Design review of the part built by this model. Coordinates are the model's own, in mm. Face numbers are marked on the shaded views. Round coordinates to 2 decimals unless told otherwise and drop trailing zeros. Order: outer loops, then holes, each group sorted by start corner. A loop starts at its lowest first (then second) coordinate and runs counter-clockwise, first axis right, second up. Notation, with made-up numbers: M 35.25,50 L 92.25,50 A18 cw 92.25,54 Z; hole C -6,6.25 d4. An arc over 180 degrees is marked long. Write each question's results on one line, items separated by ' | '. Start each with the question number.
Item 1: Take a section at B-B, the plane y = 20. Write out the cut boundary in (x, z).
Item 2: Take a section at A-A, the plane x = 0. Write out the cut boundary in (y, z), plus the area to 3 significant figures.
Item 3: Clearance check with flat-ended pins moving along their axes: pin 1 (2 mm diameter, centred on y = 40.5, z = 7.5, fed in from +X); pin 2 (1.9 mm diameter, centred on x = 6.23, y = 33.21, fed in from -Z); pin 3 (3.5 mm diameter, centred on x = -4.33, y = 27.5, fed in from -Z); pin 4 (6 mm diameter, centred on y = 7.5, z = 6, fed in from +X). State where each tip first meets the part, or that it passes through.
Item 4: The part is to be moulded in two halves that separate along Z. For the marked faces 1, 2 and 3, say which applies: +Z half, -Z half, draft (parallel to the pull), parting line (faces both ways), or undercut.
Item 5: Wall thickness on line 1 (Y direction, x = -4, z = 3); line 2 (Y direction, x = 0, z = 5.05); line 3 (Z direction, x = 21.5, y = 20.5): over which ranges is each line inside the solid? List them lowest first. Write a range as [from, to].
Item 6: Take a section at C-C, the plane z = 12.25. Write out the cut boundary in (x, y), plus the area to 3 significant figures.
Item 7: Take a section at D-D, the plane y = 36. Count the separate pieces of the cut face and the enclosed holes in it, plus the area to 3 significant figures.
```python
from build123d import *

# Parameters (mm, degrees)
SKETCH_1_R               = 27.5
EXTRUDE_1_DEPTH          = 6
SKETCH_2_R               = 6
SKETCH_2_R_2             = 3.499999999999999
EXTRUDE_2_DEPTH          = 6
PATTERN_CIRCULAR_3_COUNT = 3
CUT_EXTRUDE_1_DEPTH      = 61.37176492367935
FILLET_1_R               = 10
SKETCH_6_R               = 1.6000000000000016
SKETCH_6_R_2             = 1.6
CUT_EXTRUDE_2_DEPTH      = 62.79603560803595
SKETCH_7_R               = 2.999999999999999
CUT_EXTRUDE_3_DEPTH      = 61.37176506339406
PATTERN_CIRCULAR_4_COUNT = 3
SKETCH_8_R               = 1.5000000000000009
SKETCH_8_R_2             = 1.5000000000000018
SKETCH_8_R_3             = 1.5
CUT_EXTRUDE_4_DEPTH      = 61.37176506339406
FILLET_2_R               = 1


with BuildPart() as part:
    # 草图1 → 凸台-拉伸1 (new body)
    with BuildSketch(Plane.XY):
        with Locations((0, 25)):
            Circle(SKETCH_1_R)
    extrude(amount=EXTRUDE_1_DEPTH)

    # 草图2 → 凸台-拉伸2 (add)
    with BuildSketch(Plane(origin=(0, 0, 0), x_dir=(1, 0, 0), z_dir=(0, 1, 0))):
        with Locations((0, -11.5)):
            Circle(SKETCH_2_R)
        with Locations(Location((0, -11.5, 0), (0, 0, 270))):
            Circle(SKETCH_2_R_2, mode=Mode.SUBTRACT)
    extrude_2 = extrude(amount=EXTRUDE_2_DEPTH)

    # 阵列(圆周)3: 凸台-拉伸2 ×3 about axis
    pattern_circular_3_axis = Axis((8.33e-15, 25.000000000000004, 0), (0, 0, 1))
    for i in range(1, PATTERN_CIRCULAR_3_COUNT):
        add(extrude_2.rotate(pattern_circular_3_axis, i * 360 / PATTERN_CIRCULAR_3_COUNT))

    # 草图5 → 切除-拉伸1 (cut, through all)
    with BuildSketch(Plane.XY.offset(6)):
        with BuildLine():
            Line((-20.45167721378295, 39.57665596572934), (-15.92241547591627, 47.42156741649214))
            ThreePointArc((-15.922415475916265, 47.421567416492145), (-23.815698604072065, 38.75), (-27.378854713305756, 27.578432583507904))
            Line((-27.378854713305753, 27.578432583507908), (-22.8495929754393, 35.423344034270315))
            Line((-22.849592975439244, 35.42334403427027), (-20.451677213782926, 39.57665596572932))
        make_face()
        with BuildLine():
            Line((-2.3979157616563604, 0), (-11.456439237389594, 0))
            ThreePointArc((-11.456439237389615, 7.11e-15), (-5.05e-15, -2.5), (11.456439237389606, 3.55e-15))
            Line((11.456439237389601, 0), (2.3979157616563604, 0))
            Line((2.397915761656361, 0), (-2.397915761656361, 0))
        make_face()
        with BuildLine():
            ThreePointArc((27.378854713305756, 27.578432583507883), (23.815698604072058, 38.75000000000001), (15.922415475916232, 47.42156741649217))
            Line((15.922415475916235, 47.421567416492174), (20.451677213782762, 39.576655965729636))
            Line((20.451677213782723, 39.576655965729614), (22.8495929754391, 35.42334403427059))
            Line((22.849592975439123, 35.423344034270606), (27.378854713305756, 27.578432583507883))
        make_face()
    extrude(amount=-CUT_EXTRUDE_1_DEPTH, mode=Mode.SUBTRACT)

    # 圆角1
    fillet_1_edges = [part.edges().sort_by_distance(p)[0] for p in [
        (-17.853601002429457, 38.076655965729536, 6),
        (-20.25151676408582, 33.92334403427051, 6),
        (20.251516764085842, 33.92334403427047, 6),
        (17.853601002429485, 38.076655965729515, 6),
        (-2.3979157616563596, 3, 6),
        (2.3979157616563596, 3, 6),
    ]]
    fillet(fillet_1_edges, radius=FILLET_1_R)

    # 草图6 → 切除-拉伸2 (cut, through all)
    with BuildSketch(Plane(origin=(0, 0, 0), x_dir=(-1, 0, 0), z_dir=(0, 0, -1))):
        with Locations((-11.5, 3.5)):
            Circle(SKETCH_6_R)
        with Locations((11.5, 3.5)):
            Circle(SKETCH_6_R)
        with Locations((-4.000000000000002, 15.5)):
            Circle(SKETCH_6_R_2)
        with Locations((3.9999999999999982, 15.5)):
            Circle(SKETCH_6_R_2)
    cut_extrude_2 = extrude(amount=-CUT_EXTRUDE_2_DEPTH, mode=Mode.SUBTRACT)

    # 草图7 → 切除-拉伸3 (cut, through all)
    with BuildSketch(Plane.XY.offset(6)):
        with Locations((-11.5, 3.5)):
            Circle(SKETCH_7_R)
        with Locations((11.5, 3.5)):
            Circle(SKETCH_7_R)
    cut_extrude_3 = extrude(amount=CUT_EXTRUDE_3_DEPTH, mode=Mode.SUBTRACT)

    # 阵列(圆周)4: 切除-拉伸2, 切除-拉伸3 ×3 about axis
    pattern_circular_4_axis = Axis((0, 25.00000000000001, 0), (0, 0, 1))
    add([cut_extrude_2.rotate(pattern_circular_4_axis, i * 360 / PATTERN_CIRCULAR_4_COUNT) for i in range(1, PATTERN_CIRCULAR_4_COUNT)], mode=Mode.SUBTRACT)
    add([cut_extrude_3.rotate(pattern_circular_4_axis, i * 360 / PATTERN_CIRCULAR_4_COUNT) for i in range(1, PATTERN_CIRCULAR_4_COUNT)], mode=Mode.SUBTRACT)

    # 草图8 → 切除-拉伸4 (cut, through all)
    with BuildSketch(Plane.XY.offset(6)):
        with Locations((0, 20)):
            Circle(SKETCH_8_R)
        with Locations((-4.330127018922196, 27.500000000000004)):
            Circle(SKETCH_8_R_2)
        with Locations((4.330127018922196, 27.5)):
            Circle(SKETCH_8_R_3)
    extrude(amount=-CUT_EXTRUDE_4_DEPTH, mode=Mode.SUBTRACT)

    # 圆角2
    fillet_2_edges = [part.edges().sort_by_distance(p)[0] for p in [
        (-1.5000000000000009, 20, 0),
        (-5.830127018922198, 27.500000000000004, 0),
        (2.8301270189221963, 27.5, 0),
    ]]
    fillet(fillet_2_edges, radius=FILLET_2_R)


solid = part.part
```
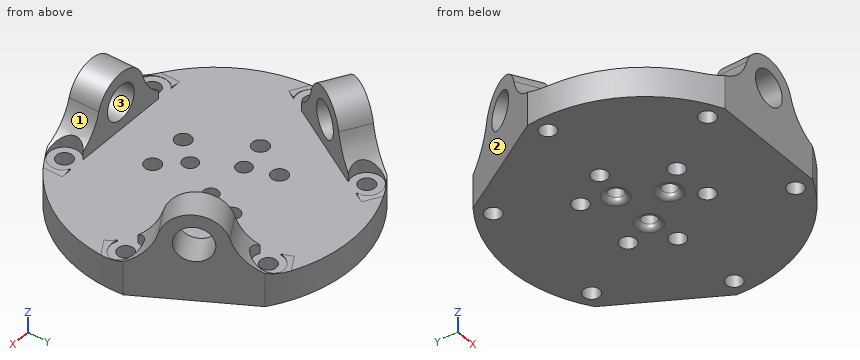
Results list:
1) outline: M -27.04,0 L -2.5,0 A1 ccw -1.5,1 L -1.5,6 L -27.04,6 Z; M 1.5,1 A1 ccw 2.5,0 L 27.04,0 L 27.04,6 L 1.5,6 Z
2) outline: M 0,0 L 17.5,0 A1 ccw 18.5,1 L 18.5,6 L 6,6 L 6,8 L 0,8 Z; M 0,15 L 6,15 L 6,17.5 L 0,17.5 Z; M 21.5,1 A1 ccw 22.5,0 L 52.5,0 L 52.5,6 L 21.5,6 Z | area: 324 mm²
3) pin 1: x = 20.5 | pin 2: through | pin 3: z = 0.34 | pin 4: x = 23.37
4) face 1: +Z half | face 2: draft | face 3: undercut
5) line 1: [0, 13.9], [17.1, 26.04], [28.96, 52.21] | line 2: [0, 18.5], [21.5, 52.5] | line 3: [0, 6]
6) outline: M -24.69,32.23 L -19.5,29.23 L -18.16,31.54 L -23.36,34.54 Z; M -19.94,40.46 L -14.75,37.46 L -13.41,39.77 L -18.61,42.77 Z; M -6.08,0 L -3.42,0 L -3.42,6 L -6.08,6 Z; M 3.42,0 L 6.08,0 L 6.08,6 L 3.42,6 Z; M 13.41,39.77 L 14.75,37.46 L 19.94,40.46 L 18.61,42.77 Z; M 18.16,31.54 L 19.5,29.23 L 24.69,32.23 L 23.36,34.54 Z | area: 95.9 mm²
7) separate pieces: 3 | enclosed holes: 0 | area: 336 mm²
